Geometry: final body of the model. Coordinates: model frame, mm. Face numbers are marked on the shaded views. A direction names the side the tool comes from. Coordinates: 2 decimals unless noted, no trailing zeros. Write each loop counter-clockwise with the first axis right and the second up, starting at its lowest first coordinate (ties: lowest second). Pieces come first, ordered by that corner, then holes. Notation, with made-up numbers: (26, -3) - (54, -3) arc R26 cw to (54, 29) - close; hole circle Ø2 at (19.25, 20.5). An arc over 180 degrees is marked (long way). Answer as a JSON object with one key per item and string values. Group by question number.
Item 1: First-contact query: pin 1 Ø2 at (x, y) = (-15, 2.5) entering from -Z; pin 2 Ø3 at (x, y) = (-11, -3.5) entering from +Z; pin 3 Ø5 at (x, y) = (-7.5, 0) entering from -Z; pin 4 Ø5 at (x, z) = (0.5, 48) entering from -Y. Flat tips, straight axial feed; report the tip coordinate or a pass-through.
Item 2: Mould query, pull axis Z, two halves, no side actions, for the marked faces 4, 5 and 6. Classes: pulls with the +Z half, pulls with the -Z half, needs draft (parallel to the pull), parting line crosses it, or undercut.
Item 3: Section A-A on x = -7. Return loops of the section in (y, z), and give its area (3 significant figures).
Item 4: Line query: line 1 along X through (y, z) = (0.75, 49.25); line 2 along X through (y, z) = (-1.25, 45.5); line 3 along X through (y, z) = (-1.75, 46.5). Output: solid intervals per line, ascending. Write a range as from..to.
Item 5: Set-up query: the marked faces 1, 2 and 3. Return all of +Z, -Z, +X, -X, +Y, -Y with unobstructed straight access to the full face (end or side cutting, diameter ignored); none if empty.
Item 6: Section B-B on x = 6. Return loops of the section in (y, z), and give its area (3 significant figures).
```python
from build123d import *

# Parameters (mm, degrees)
EXTRUDE_1_DEPTH = 4.9
CHAMFER_1_SIZE  = 1


with BuildPart() as part:
    # Эскиз2 → Бобышка-Вытянуть1 (new, symmetric)
    with BuildSketch(Plane(origin=(0, 0, 0), x_dir=(1, 0, 0), z_dir=(0, 1, 0))):
        with BuildLine():
            Line((-19.066440629, -51.056055877), (-18.366754734, -49.182439148))
            ThreePointArc((-18.366754734, -49.182439148), (-16.897260285, -49.706464317), (-15.412844037, -50.186594213))
            Line((-15.412844037, -50.186594213), (-14.972477064, -48.752691521))
            Line((-14.972477064, -48.752691521), (-14.913761468, -48.561504496))
            ThreePointArc((-14.913761468, -48.561504496), (-15.200281945, -48.472584301), (-15.486272306, -48.381973607))
            Line((-15.486272306, -48.381973607), (-15.181424426, -47.429572551))
            Line((-15.181424426, -47.429572551), (-14.620183486, -47.605569368))
            Line((-14.620183486, -47.605569368), (-12.098110765, -45.366305195))
            ThreePointArc((-12.098110765, -45.366305195), (-10.925741151, -45.252992376), (-10.458715596, -46.334277464))
            Line((-10.458715596, -46.334277464), (-11.229357798, -49.748382119))
            Line((-11.229357798, -49.748382119), (-11.559633028, -51.211569828))
            ThreePointArc((-11.559633028, -51.211569828), (0, -52.5), (11.559633028, -51.211569828))
            Line((11.559633028, -51.211569828), (11.229357798, -49.748382119))
            Line((11.229357798, -49.748382119), (10.458715596, -46.334277464))
            ThreePointArc((10.458715596, -46.334277464), (10.925741151, -45.252992376), (12.098110765, -45.366305195))
            Line((12.098110765, -45.366305195), (14.620183486, -47.605569368))
            Line((14.620183486, -47.605569368), (15.181424426, -47.429572551))
            Line((15.181424426, -47.429572551), (15.486272306, -48.381973607))
            ThreePointArc((15.486272306, -48.381973607), (15.200281945, -48.472584301), (14.913761468, -48.561504496))
            Line((14.913761468, -48.561504496), (14.972477064, -48.752691521))
            Line((14.972477064, -48.752691521), (15.412844037, -50.186594213))
            ThreePointArc((15.412844037, -50.186594213), (16.897260285, -49.706464317), (18.366754734, -49.182439148))
            Line((18.366754734, -49.182439148), (19.066440629, -51.056055877))
            ThreePointArc((19.066440629, -51.056055877), (17.189479987, -51.718195809), (15.289593803, -52.311359391))
            Line((15.289593803, -52.311359391), (14.089034129, -48.203800394))
            Line((14.089034129, -48.203800394), (11.566961408, -45.964536221))
            ThreePointArc((11.566961408, -45.964536221), (11.332487486, -45.941873657), (11.239082375, -46.158130675))
            Line((11.239082375, -46.158130675), (12.009724576, -49.57223533))
            Line((12.009724576, -49.57223533), (12.8323427, -52.967735281))
            ThreePointArc((12.8323427, -52.967735281), (0, -54.5), (-12.8323427, -52.967735281))
            Line((-12.8323427, -52.967735281), (-12.009724576, -49.57223533))
            Line((-12.009724576, -49.57223533), (-11.239082375, -46.158130675))
            ThreePointArc((-11.239082375, -46.158130675), (-11.332487486, -45.941873657), (-11.566961408, -45.964536221))
            Line((-11.566961408, -45.964536221), (-14.089034129, -48.203800394))
            Line((-14.089034129, -48.203800394), (-15.289593803, -52.311359391))
            ThreePointArc((-15.289593803, -52.311359391), (-17.189479987, -51.718195809), (-19.066440629, -51.056055877))
        make_face()
    extrude(amount=EXTRUDE_1_DEPTH, both=True)

    # Фаска1
    # the kernel refuses this chamfer: 1 mm, written as the material it takes off along each edge
    with BuildSketch(Plane(origin=(-18.366754734, 7.496724976, 49.182439148), x_dir=(0.9401293921516592, 0, 0.3408177313646573), z_dir=(0, -1, 0))) as chamfer_1_piece_1:
        with BuildLine():
            Line((1.009757262, 0), (-CHAMFER_1_SIZE * 0.00961673582767, CHAMFER_1_SIZE * 0.999953758127))
            Line((-CHAMFER_1_SIZE * 0.00961673582767, CHAMFER_1_SIZE * 0.999953758127), (0, 0))
            ThreePointArc((0, 0), (0.519160584, 0.002425756), (1.009757262, 0))
        make_face()
    extrude(amount=14.993449951, mode=Mode.SUBTRACT)
    with BuildSketch(Plane(origin=(18.366754734, 7.496724976, 49.182439148), x_dir=(0.34984294732251126, 0, 0.9368083647196467), z_dir=(0, -1, 0))) as chamfer_1_piece_2:
        with BuildLine():
            Line((CHAMFER_1_SIZE, 0), (-0.009710569, 1.009710569))
            ThreePointArc((-0.009710569, 1.009710569), (-0.002566987, 0.519159905), (0, 0))
            Line((0, 0), (CHAMFER_1_SIZE, 0))
        make_face()
    extrude(amount=14.993449951, mode=Mode.SUBTRACT)
    with BuildSketch(Plane(origin=(15.289593803, 7.471682988, 52.311359391), x_dir=(-0.2805430055685125, 0, -0.9598414567138605), z_dir=(0, -1, 0))) as chamfer_1_piece_3:
        with BuildLine():
            Line((CHAMFER_1_SIZE, 0), (0.009010472, 0.990989528))
            ThreePointArc((0.009010472, 0.990989528), (0.002381843, 0.509524531), (0, 0))
            Line((0, 0), (CHAMFER_1_SIZE, 0))
        make_face()
    extrude(amount=14.943365976, mode=Mode.SUBTRACT)
    with BuildSketch(Plane(origin=(12.8323427, 7.471682988, 52.967735281), x_dir=(-0.9739856496022864, 0, 0.22660969610502585), z_dir=(0, -1, 0)), Plane(origin=(-15.289593803, 7.471682988, 52.311359391), x_dir=(-0.9572510798876259, 0, -0.2892583102591421), z_dir=(0, -1, 0))) as chamfer_1_piece_4:
        with BuildLine():
            Line((0.991030491, 0), (CHAMFER_1_SIZE * 0.00909202285035, CHAMFER_1_SIZE * 0.999958666706))
            Line((CHAMFER_1_SIZE * 0.00909202285035, CHAMFER_1_SIZE * 0.999958666706), (0, 0))
            ThreePointArc((0, 0), (0.509525126, -0.002250864), (0.991030491, 0))
        make_face()
    extrude(amount=14.943365976, mode=Mode.SUBTRACT)
    with BuildSketch(Plane(origin=(-12.8323427, -7.471682988, 52.967735281), x_dir=(0.23545582936194254, 0, -0.9718850510320034), z_dir=(0, 1, 0))) as chamfer_1_piece_5:
        with BuildLine():
            Line((CHAMFER_1_SIZE, 0), (0.009010472, -0.990989528))
            ThreePointArc((0.009010472, -0.990989528), (0.002381843, -0.509524531), (0, 0))
            Line((0, 0), (CHAMFER_1_SIZE, 0))
        make_face()
    extrude(amount=14.943365976, mode=Mode.SUBTRACT)


solid = part.part
```
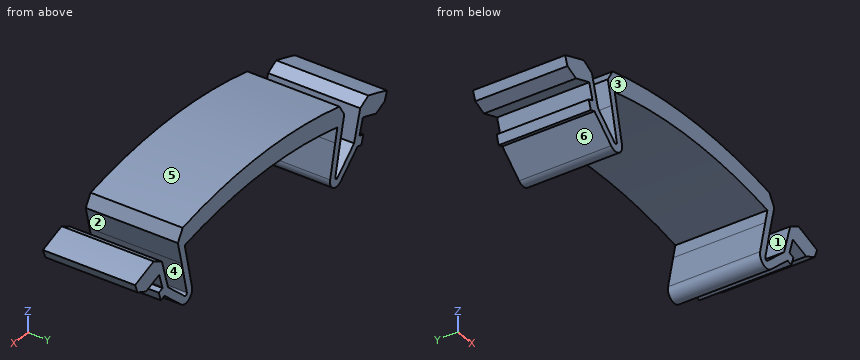
Checks:
{
 "1": {"pin 1": "z = 47.05", "pin 2": "z = 53.67", "pin 3": "z = 51.54", "pin 4": "through"},
 "2": {"face 4": "undercut", "face 5": "pulls with the +Z half", "face 6": "pulls with the -Z half"},
 "3": {"outline": "(-4.9, 52.03) - (4.9, 52.03) - (4.9, 54.05) - (-4.9, 54.05) - close", "area": "19.8 mm^2"},
 "4": {"line 1": "-15.13..-14.39, -11.94..-11.12, 11.12..11.94, 14.39..15.13", "line 2": "-12.25..-10.64, 10.64..12.25", "line 3": "-13.37..-12.17, -11.32..-10.5, 10.5..11.32, 12.17..13.37"},
 "5": {"face 1": "+Z, +Y, -Y", "face 2": "+Y, -Y", "face 3": "+Z, -Z, +X, -X, -Y"},
 "6": {"outline": "(-4.9, 52.16) - (4.9, 52.16) - (4.9, 54.17) - (-4.9, 54.17) - close", "area": "19.7 mm^2"}
}
